Autodesk Inventor part; units mm, degrees
ref_plane "Arbeitsebene1" through (0, 0, 0) normal (1, 0, 0) x (0, 1, 0)
ref_plane "Arbeitsebene2" through (0, 0, -2.5) normal (0, 0, 1) x (1, 0, 0)
ref_plane "Arbeitsebene3" through (0, 0, 0) normal (0, 1, 0) x (-1, 0, 0)
sketch "Skizze2" plane through (0, 0, 0) normal (0, 1, 0) x (-1, 0, 0)
  line L0 (0, 0) -> (14.5, 0)
  line L1 (14.5, 0) -> (14.5, -35.5)
  line L2 (14.5, -35.5) -> (0, -35.5)
  line L3 (0, -35.5) -> (0, 0)
  dimension "d2" = 29
  dimension "d3" = 35.5
revolve "Umdrehung1" add sketch "Skizze2" angle 360 about axis through (0, 0, -35.5) along (0, 0, 1)
ref_plane "Arbeitsebene1" through (0, 0, 0) normal (1, 0, 0) x (0, 1, 0)
ref_plane "Arbeitsebene2" through (0, 0, -2.5) normal (0, 0, 1) x (1, 0, 0)
sketch "Skizze4" plane through (0, 0, -2.5) normal (0, 0, 1) x (1, 0, 0)
  line L0 (25, -25) -> (-25, -25)
  line L1 (-25, -25) -> (-25, 25)
  line L2 (-25, 25) -> (25, 25)
  line L3 (25, 25) -> (25, -25)
  line L4 (25, -25) -> (-25, 25) construction
  line L5 (-25, -25) -> (25, 25) construction
  point P0 (0, 0)
  dimension "d7" = 50
  dimension "d8" = 50
extrude "Extrusion1" add sketch "Skizze4" against normal blind 5
ref_plane "Arbeitsebene3" through (0, 0, 0) normal (0, 1, 0) x (-1, 0, 0)
sketch "Skizze5" plane through (0, 0, 0) normal (0, 1, 0) x (-1, 0, 0)
  line L0 (14.5, -2.5) -> (14.5, 0)
  line L1 (14.5, -35.5) -> (14.5, -7.5)
  line L2 (14.5, -9.5) -> (22, -9.5)
  line L3 (22, -9.5) -> (22, -10.5)
  line L4 (22, -10.5) -> (14.5, -10.5)
  line L5 (25, -2.5) -> (-25, -2.5)
  line L6 (25, -2.5) -> (25, -7.5)
  line L7 (-25, -7.5) -> (25, -7.5)
  line L8 (-25, -2.5) -> (-25, -7.5)
  line L9 (0, 0) -> (0, -35.5)
  line L10 (14.5, -9.5) -> (14.5, -10.5)
  line L11 (14.5, -11.5) -> (22, -11.5)
  line L12 (22, -11.5) -> (22, -12.5)
  line L13 (22, -12.5) -> (14.5, -12.5)
  line L14 (14.5, -11.5) -> (14.5, -12.5)
  line L15 (14.5, -13.5) -> (22, -13.5)
  line L16 (22, -13.5) -> (22, -14.5)
  line L17 (22, -14.5) -> (14.5, -14.5)
  line L18 (14.5, -13.5) -> (14.5, -14.5)
  line L19 (14.5, -15.5) -> (22, -15.5)
  line L20 (22, -15.5) -> (22, -16.5)
  line L21 (22, -16.5) -> (14.5, -16.5)
  line L22 (14.5, -15.5) -> (14.5, -16.5)
  line L23 (14.5, -17.5) -> (22, -17.5)
  line L24 (22, -17.5) -> (22, -18.5)
  line L25 (22, -18.5) -> (14.5, -18.5)
  line L26 (14.5, -17.5) -> (14.5, -18.5)
  line L27 (14.5, -19.5) -> (22, -19.5)
  line L28 (22, -19.5) -> (22, -20.5)
  line L29 (22, -20.5) -> (14.5, -20.5)
  line L30 (14.5, -19.5) -> (14.5, -20.5)
  line L31 (14.5, -21.5) -> (22, -21.5)
  line L32 (22, -21.5) -> (22, -22.5)
  line L33 (22, -22.5) -> (14.5, -22.5)
  line L34 (14.5, -21.5) -> (14.5, -22.5)
  line L35 (14.5, -23.5) -> (22, -23.5)
  line L36 (22, -23.5) -> (22, -24.5)
  line L37 (22, -24.5) -> (14.5, -24.5)
  line L38 (14.5, -23.5) -> (14.5, -24.5)
  point P0 (22, -10)
  point P1 (18.25, -13.5)
  point P2 (18.25, -22.5)
  dimension "d12" = 1
  dimension "d13" = 2
  dimension "d14" = 44
  dimension "d15" = 1
  dimension "d16" = 1
  dimension "d17" = 1
  dimension "d18" = 1
  dimension "d19" = 1
  dimension "d20" = 1
  dimension "d21" = 1
  dimension "d22" = 1
  dimension "d23" = 1
  dimension "d24" = 1
  dimension "d25" = 1
  dimension "d26" = 1
  dimension "d27" = 1
  dimension "d28" = 1
  dimension "d29" = 44
revolve "Umdrehung2" add sketch "Skizze5" angle 360 about axis through (0, 0, 0) along (0, 0, -1) contours L1 L2 L3 L4 | L1 L11 L12 L13 | L1 L15 L16 L17 | L1 L19 L20 L21 | L1 L23 L24 L25 | L1 L27 L28 L29 | L1 L31 L32 L33 | L1 L35 L36 L37
ref_plane "Arbeitsebene4" through (0, 0, -35.5) normal (0, 0, -1) x (-1, 0, 0)
sketch "Skizze6" plane through (0, 0, -35.5) normal (0, 0, -1) x (-1, 0, 0)
  line L0 (-25, 25) -> (25, 25)
  line L1 (25, 25) -> (25, -25)
  line L2 (25, -25) -> (-25, -25)
  line L3 (-25, -25) -> (-25, 25)
  line L4 (-25, 25) -> (25, -25) construction
  line L5 (25, 25) -> (-25, -25) construction
  point P0 (0, 0)
  dimension "d32" = 50
  dimension "d33" = 50
extrude "Extrusion2" add sketch "Skizze6" against normal blind 7
sketch "Skizze7" plane through (25, -25, -35.5) normal (0, 0, -1) x (-1, 0, 0)
  point P0 (25, 25)
  point P1 (25, 25)
hole "Bohrung1" at (0, 0, -35.5) direction (0, 0, 1) diameter 27 depth 35.5
sketch "Skizze8" plane through (25, -25, -35.5) normal (0, 0, -1) x (-1, 0, 0)
  line L0 (0, 0) -> (50, 0)
  line L1 (25, 0) -> (25, 50) construction
  line L2 (50, 50) -> (0, 50)
  line L3 (50, 50) -> (50, 0)
  line L4 (50, 25) -> (0, 25) construction
  line L5 (0, 0) -> (0, 50)
  point P0 (25, 25)
  point P1 (46.124, 3.876)
  point P2 (3.876, 3.876)
  point P3 (46.124, 46.124)
  point P4 (3.876, 46.124)
  dimension "d75" = 42.248
  dimension "d76" = 42.248
hole "Bohrung2" at (-21.124, -21.124, -35.5) at (21.124, -21.124, -35.5) at (-21.124, 21.124, -35.5) at (21.124, 21.124, -35.5) direction (0, 0, 1) diameter 5 depth 7
sketch "Skizze9" plane through (0, 0, -2.5) normal (0, 0, 1) x (1, 0, 0)
  line L0 (25, 25) -> (25, -25)
  line L1 (25, 0) -> (-25, 0) construction
  line L2 (-25, -25) -> (-25, 25)
  line L3 (-25, 25) -> (25, 25)
  line L4 (0, 25) -> (0, -36.4207) construction
  point P0 (0, 0)
  point P1 (-21.124, 21.124)
  point P2 (21.124, 21.124)
  point P3 (-21.124, -21.124)
  point P4 (21.124, -21.124)
  dimension "d73" = 42.248
  dimension "d74" = 42.248
hole "Bohrung3" at (-21.124, 21.124, -2.5) at (21.124, 21.124, -2.5) at (-21.124, -21.124, -2.5) at (21.124, -21.124, -2.5) direction (0, 0, -1) diameter 5 depth 5
equation "\"d16\" = d15"
equation "\"d17\" = d15"
equation "\"d18\" = d15"
equation "\"d26\" = d22"
equation "\"d27\" = d22"
properties part number "cylinder" material "Bronze, Guss"
For this review, take the finished solid that the model builds, in its own axes (mm). A direction names the side the tool comes from. Round coordinates to 2 decimals unless told otherwise and drop trailing zeros. Loops run counter-clockwise (first coordinate to the right, second up) from the corner with the lowest first, then second, coordinate; pieces in that order, holes last. Notation, with made-up numbers: (-7, -10) - (24, -10) arc R22 ccw to (24, 8) - close; hole circle Ø7 at (24, 47.25). An arc over 180 degrees is marked (long way). One line per question, with ' | ' between items.
Q1. For line 1 along Y through (x, z) = (0, -31); line 2 along X through (y, z) = (22, -30); line 3 along Z through (x, y) = (5, 23), list the stretches that pass through material, from the lowest coordinate up. Write a range as [from, to].
Taken from the geometry:
line 1: y = [-25, -13.5], [13.5, 25] | line 2: x = [-25, -23.47], [-18.78, 18.78], [23.47, 25] | line 3: z = [-35.5, -28.5], [-7.5, -2.5]
Q2. Take a section at B-B (x = -16). State how many separate pieces and enclosed holes the cut face has, and give its area (3 significant figures).
Taken from the geometry:
separate pieces: 10 | enclosed holes: 0 | area: 842 mm²
Q3. The part is to be moulded in two halves that separate along X. For faces 3 (the cylindrical face through (20.37, 18.74, -5.04)), 4 (the cylindrical face through (-6.691, -12.864, -21.007)), 5 (the flat face through (-14, -5, -16.5)), say which applies: released by +X, released by -X, zero draft, split by the parting line, or undercut.
Taken from the geometry:
face 3: undercut | face 4: split by the parting line | face 5: zero draft
Q4. Take a section at A-A (z = -5.5). Give the boundary of the cut face in (x, y).
Taken from the geometry:
outline: (-25, -25) - (25, -25) - (25, 25) - (-25, 25) - close; hole circle Ø5 at (-21.12, -21.12); hole circle Ø5 at (-21.12, 21.12); hole circle Ø27 at (0, 0); hole circle Ø5 at (21.12, -21.12); hole circle Ø5 at (21.12, 21.12)
Q5. Tool access review of faces 1 (the flat face through (-14, -5, -11.5)), 2 (the cylindrical face through (-19.6, 19.14, -31.95)): name each direction out of +Z, -Z, +X, -X, +Y, -Y from which nothing blocks a thin tool from reaching the whole face with its end or side.
Taken from the geometry:
face 1: none | face 2: +Z, -Z
Q6. For pin 1 (25 mm diameter, centred on x = -5.5, y = 8.5, fed in from +Z); pin 2 (6 mm diameter, centred on x = -21.124, y = 21.124, fed in from +Z); pin 3 (5 mm diameter, centred on y = -10, z = -16.5, fed in from +X); pin 4 (3 mm diameter, centred on y = 1.5, z = -25.5, fed in from -X), all flat-tipped, find the tip position at first contact; note any pin that passes through.
Taken from the geometry:
pin 1: stops at z = 0 | pin 2: stops at z = -2.5 | pin 3: stops at x = 20.68 | pin 4: stops at x = -22
